Check sheet for the modelled part. Datum: model origin and axes. Units: mm. Round coordinates to 2 decimals unless told otherwise and drop trailing zeros. Order: outer loops, then holes, each group sorted by start corner. A loop starts at its lowest first (then second) coordinate and runs counter-clockwise, first axis right, second up. Notation, with made-up numbers: M 9,30 L 36,30 A23 ccw 36,38 Z; hole C -27,-29.75 d10. An arc over 180 degrees is marked long. One line per item, written item: value. Start each with the question number.
(1) Cross-section at B-B, the plane y = 0.9. Count the separate pieces of the cut face and the enclosed holes in it, and give its area (3 significant figures).
(2) Thickness scan on L1, parallel to Z at x = 66.5, y = 1.6; L2, parallel to Z at x = 97, y = 0.6; L3, parallel to X at y = 1.3, z = -58. Record the ranges inside material, lowest first.
(3) Cross-section at A-A, the plane x = 34. Enter the section's corners in (y, z).
from build123d import *

# Parameters (mm, degrees)
SKETCH1_W           = 130
SKETCH1_H           = 90
BOSS_EXTRUDE2_DEPTH = 2
SKETCH2_R           = 2
CUT_EXTRUDE1_DEPTH  = 10
CUT_EXTRUDE3_DEPTH  = 10
SKETCH5_R           = 1
CUT_EXTRUDE4_DEPTH  = 10


with BuildPart() as part:
    # Sketch1 → Boss-Extrude2 (new body)
    with BuildSketch(Plane(origin=(0, 0, 0), x_dir=(1, 0, 0), z_dir=(0, 1, 0))):
        with Locations((56.787418592, 40.403463793)):
            Rectangle(SKETCH1_W, SKETCH1_H)
    extrude(amount=BOSS_EXTRUDE2_DEPTH)

    # Sketch2 → Cut-Extrude1 (cut)
    with BuildSketch(Plane(origin=(0, 2, 0), x_dir=(1, 0, 0), z_dir=(0, 1, 0))):
        with Locations(Location((16.787418592, 50.403463793, 0), (0, 0, 270))):
            Circle(SKETCH2_R)
        with Locations(Location((16.787418592, 30.403463793, 0), (0, 0, 270))):
            Circle(SKETCH2_R)
        with Locations(Location((96.787418592, 50.403463793, 0), (0, 0, 270))):
            Circle(SKETCH2_R)
        with Locations(Location((96.787418592, 30.403463793, 0), (0, 0, 270))):
            Circle(SKETCH2_R)
    extrude(amount=-CUT_EXTRUDE1_DEPTH, mode=Mode.SUBTRACT)

    # Sketch4 → Cut-Extrude3 (cut)
    with BuildSketch(Plane(origin=(0, 2, 0), x_dir=(1, 0, 0), z_dir=(0, 1, 0))):
        with BuildLine():
            Line((26.787418592, 52.903463793), (48.787418592, 52.903463793))
            ThreePointArc((48.787418592, 52.903463793), (50.287418592, 51.403463793), (48.787418592, 49.903463793))
            Line((48.787418592, 49.903463793), (26.787418592, 49.903463793))
            ThreePointArc((26.787418592, 49.903463793), (25.287418592, 51.403463793), (26.787418592, 52.903463793))
        make_face()
        with BuildLine():
            Line((26.787418592, 30.903463793), (48.787418592, 30.903463793))
            ThreePointArc((48.787418592, 30.903463793), (50.287418592, 29.403463793), (48.787418592, 27.903463793))
            Line((48.787418592, 27.903463793), (26.787418592, 27.903463793))
            ThreePointArc((26.787418592, 27.903463793), (25.287418592, 29.403463793), (26.787418592, 30.903463793))
        make_face()
        with BuildLine():
            Line((64.787418592, 52.903463793), (86.787418592, 52.903463793))
            ThreePointArc((86.787418592, 52.903463793), (88.287418592, 51.403463793), (86.787418592, 49.903463793))
            Line((86.787418592, 49.903463793), (64.787418592, 49.903463793))
            ThreePointArc((64.787418592, 49.903463793), (63.287418592, 51.403463793), (64.787418592, 52.903463793))
        make_face()
        with BuildLine():
            Line((64.787418592, 30.903463793), (86.787418592, 30.903463793))
            ThreePointArc((86.787418592, 30.903463793), (88.287418592, 29.403463793), (86.787418592, 27.903463793))
            Line((86.787418592, 27.903463793), (64.787418592, 27.903463793))
            ThreePointArc((64.787418592, 27.903463793), (63.287418592, 29.403463793), (64.787418592, 30.903463793))
        make_face()
    extrude(amount=-CUT_EXTRUDE3_DEPTH, mode=Mode.SUBTRACT)

    # Sketch5 → Cut-Extrude4 (cut)
    with BuildSketch(Plane(origin=(0, 2, 0), x_dir=(1, 0, 0), z_dir=(0, 1, 0))):
        with Locations(Location((1.287418592, 10.403463793, 0), (0, 0, 270))):
            Circle(SKETCH5_R)
        with Locations(Location((112.287418592, 10.403463793, 0), (0, 0, 270))):
            Circle(SKETCH5_R)
        with Locations(Location((84.287418592, 56.920801797, 0), (0, 0, 270))):
            Circle(SKETCH5_R)
        with Locations(Location((116.787418592, 57.403463793, 0), (0, 0, 270))):
            Circle(SKETCH5_R)
        with Locations(Location((116.787418592, 79.403463793, 0), (0, 0, 270))):
            Circle(SKETCH5_R)
        with Locations(Location((84.287418592, 79.403463793, 0), (0, 0, 270))):
            Circle(SKETCH5_R)
        with Locations(Location((-3.212581408, 57.403463793, 0), (0, 0, 270))):
            Circle(SKETCH5_R)
        with Locations(Location((29.287418592, 57.403463793, 0), (0, 0, 270))):
            Circle(SKETCH5_R)
        with Locations(Location((29.287418592, 79.403463793, 0), (0, 0, 270))):
            Circle(SKETCH5_R)
        with Locations(Location((-3.212581408, 79.403463793, 0), (0, 0, 270))):
            Circle(SKETCH5_R)
    extrude(amount=-CUT_EXTRUDE4_DEPTH, mode=Mode.SUBTRACT)


solid = part.part
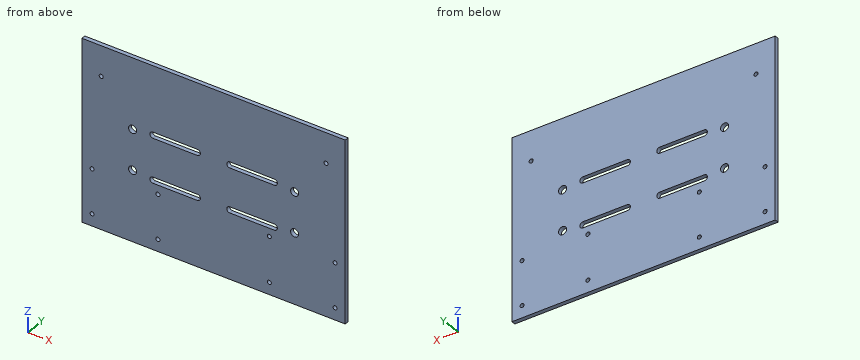
Values found:
1. separate pieces: 1
1. enclosed holes: 18
1. area: 11,300 mm^2
2. L1: -85.4 to -52.9, -49.9 to -30.9, -27.9 to 4.6
2. L2: -85.4 to -52.39, -48.41 to -32.39, -28.41 to 4.6
2. L3: -8.21 to -4.02, -2.41 to 28.48, 30.09 to 115.98, 117.59 to 121.79
3. outline: M 0,-85.4 L 2,-85.4 L 2,-52.9 L 0,-52.9 Z; M 0,-49.9 L 2,-49.9 L 2,-30.9 L 0,-30.9 Z; M 0,-27.9 L 2,-27.9 L 2,4.6 L 0,4.6 Z
